from build123d import *

# Parameters (mm, degrees)
BOSS_EXTRUDE1_DEPTH = 168.35
FILLET1_R           = 1
SKETCH2_R           = 1.8
CUT_EXTRUDE1_DEPTH  = 200
CUT_EXTRUDE2_DEPTH  = 2
LPATTERN1_COUNT     = 3
LPATTERN1_PITCH     = 116
CUT_EXTRUDE3_DEPTH  = 1


with BuildPart() as part:
    # Sketch1 → Boss-Extrude1 (new body)
    with BuildSketch(Plane.XY):
        Polygon((0, 0), (5.8, 0), (8.7, 3.9), (-2.9, 3.9), align=None)
    extrude(amount=BOSS_EXTRUDE1_DEPTH)

    # Fillet1
    fillet1_edges = [part.edges().sort_by_distance(p)[0] for p in [
        (-2.9, 3.9, 84.175),
        (8.7, 3.9, 84.175),
    ]]
    fillet(fillet1_edges, radius=FILLET1_R)

    # Sketch2 → Cut-Extrude1 (cut)
    with BuildSketch(Plane.XZ):
        with Locations(Location((2.9, 126, 0), (0, 0, 270))):
            Circle(SKETCH2_R)
    cut_extrude1 = extrude(amount=-CUT_EXTRUDE1_DEPTH, mode=Mode.SUBTRACT)

    # Sketch3 → Cut-Extrude2 (cut)
    with BuildSketch(Plane.XZ):
        Polygon((2.902268292, 122.651369207), (5.80113348, 124.327649002), (5.798865189, 127.676279795), (2.897731708, 129.348630793), (-0.00113348, 127.672350998), (0.001134811, 124.323720205), align=None)
    cut_extrude2 = extrude(amount=-CUT_EXTRUDE2_DEPTH, mode=Mode.SUBTRACT)

    # LPattern1: Cut-Extrude1, Cut-Extrude2 ×3
    with Locations(*[(0, 0, -i * LPATTERN1_PITCH) for i in range(1, LPATTERN1_COUNT)]):
        add(cut_extrude1, mode=Mode.SUBTRACT)
        add(cut_extrude2, mode=Mode.SUBTRACT)

    # Sketch4 → Cut-Extrude3 (cut)
    with BuildSketch(Plane(origin=(0, 3.9, 0), x_dir=(1, 0, 0), z_dir=(0, 1, 0))):
        with BuildLine():
            Line((5.439754142, -74.65), (5.439754142, -75.626923077))
            Line((5.439754142, -75.626923077), (2.199880343, -75.626923077))
            Line((2.199880343, -75.626923077), (1.686614118, -78.132196514))
            add(Edge.make_bspline(
                [(1.686614118, -78.132196514), (1.787459033, -78.10435556), (1.982830106, -78.050418115), (2.271192299, -77.990530983), (2.544946796, -77.954430025), (2.722589054, -77.949500672), (2.808549214, -77.947115385)],
                knots=[0, 0, 0, 0, 1.100273476, 2.13160584, 3.095893838, 4, 4, 4, 4], degree=3))
            add(Edge.make_bspline(
                [(2.808549214, -77.947115385), (2.91491282, -77.949417538), (3.124050244, -77.953944147), (3.430044807, -77.997410395), (3.722143609, -78.065826877), (3.999735773, -78.161404868), (4.263334843, -78.283623499), (4.510515564, -78.43629548), (4.74498817, -78.614639759), (4.96254623, -78.819685828), (5.159915954, -79.045351085), (5.33345054, -79.287987862), (5.480850161, -79.545238143), (5.599397644, -79.819559799), (5.694060725, -80.107920067), (5.757067225, -80.413353024), (5.799022697, -80.732979693), (5.803710049, -80.951522845), (5.806100295, -81.062965745)],
                knots=[0, 0, 0, 0, 1.052922333, 2.070308379, 3.05430497, 4.020497103, 4.973039431, 5.925935799, 6.892292201, 7.88610001, 8.88166317, 9.857072816, 10.836096531, 11.812156883, 12.81219415, 13.836441305, 14.89672472, 16, 16, 16, 16], degree=3))
            add(Edge.make_bspline(
                [(5.806100295, -81.062965745), (5.804290341, -81.140586931), (5.800694891, -81.294780318), (5.782410734, -81.52377275), (5.747207107, -81.747917317), (5.699942087, -81.967243755), (5.638594506, -82.181336832), (5.564329295, -82.390809347), (5.473444392, -82.594357527), (5.373754721, -82.793907352), (5.261505377, -82.984947575), (5.136922439, -83.163606603), (5.005299209, -83.332564541), (4.863672296, -83.490009343), (4.710725302, -83.634906413), (4.548310535, -83.768115664), (4.377723993, -83.891889856), (4.196326512, -84.00120473), (4.008160183, -84.101796775), (3.810507678, -84.184320116), (3.6078682, -84.258099482), (3.397325217, -84.316908268), (3.179355627, -84.362989005), (2.953600131, -84.394287068), (2.721242736, -84.417082945), (2.563740024, -84.418509945), (2.484180223, -84.419230769)],
                knots=[0, 0, 0, 0, 1.056347294, 2.098418968, 3.122841568, 4.141288669, 5.149314143, 6.15115421, 7.162517403, 8.180376062, 9.185164535, 10.17417709, 11.141909838, 12.097768115, 13.052685741, 14.0056014, 14.954263652, 15.917497458, 16.885230207, 17.854509472, 18.828990115, 19.81800267, 20.826176721, 21.857883937, 22.917946725, 24, 24, 24, 24], degree=3))
            add(Edge.make_bspline(
                [(2.484180223, -84.419230769), (2.389272632, -84.417350703), (2.202553157, -84.413651895), (1.928993613, -84.374957303), (1.665791722, -84.319538359), (1.415066233, -84.236163939), (1.174570151, -84.131695658), (0.947541183, -83.999662363), (0.728178321, -83.850040659), (0.525399135, -83.673473413), (0.337195712, -83.48048145), (0.16872157, -83.271046726), (0.018679479, -83.048625887), (-0.110527818, -82.812138768), (-0.22074029, -82.562206766), (-0.307322508, -82.297893456), (-0.377204317, -82.020579874), (-0.40676834, -81.829662107), (-0.42178432, -81.732692308)],
                knots=[0, 0, 0, 0, 1.0467383, 2.05933395, 3.04377827, 4.011590433, 4.970194871, 5.932262533, 6.905835911, 7.896367577, 8.894135286, 9.877477877, 10.858688626, 11.851381753, 12.8477658, 13.868841284, 14.917554742, 16, 16, 16, 16], degree=3))
            Line((-0.42178432, -81.732692308), (0.433023372, -81.732692308))
            add(Edge.make_bspline(
                [(0.433023372, -81.732692308), (0.454056089, -81.823523939), (0.494482139, -81.998107378), (0.583216355, -82.243393385), (0.691708488, -82.461976416), (0.820716036, -82.656747924), (0.974612905, -82.826589553), (1.150225136, -82.977947414), (1.347114297, -83.114495445), (1.565898729, -83.228313118), (1.796711466, -83.325383083), (2.038285088, -83.390021624), (2.284041916, -83.435471911), (2.450262338, -83.440021489), (2.533789598, -83.442307692)],
                knots=[0, 0, 0, 0, 1.136247022, 2.183929868, 3.172523383, 4.106158343, 5.02341133, 5.958108904, 6.928429099, 7.938127109, 8.96079061, 9.975095812, 10.982467395, 12, 12, 12, 12], degree=3))
            add(Edge.make_bspline(
                [(2.533789598, -83.442307692), (2.615319365, -83.440074004), (2.775852142, -83.435675853), (3.01210313, -83.40182397), (3.240193881, -83.349688008), (3.457873759, -83.271665046), (3.668951949, -83.176837633), (3.868089138, -83.055148749), (4.061046254, -82.915103984), (4.241825675, -82.754657727), (4.40739589, -82.577847343), (4.553689334, -82.38876958), (4.675546506, -82.187065876), (4.778237188, -81.976228224), (4.856215094, -81.753945865), (4.911843764, -81.521260524), (4.944509231, -81.277597471), (4.9490028, -81.111401706), (4.951292603, -81.02671274)],
                knots=[0, 0, 0, 0, 1.027316725, 2.022795036, 3.002884548, 3.971462791, 4.93288096, 5.914575861, 6.907176829, 7.935150275, 8.956128384, 9.956726525, 10.942570165, 11.921478529, 12.907843606, 13.90538589, 14.932640048, 16, 16, 16, 16], degree=3))
            add(Edge.make_bspline(
                [(4.951292603, -81.02671274), (4.949500598, -80.950306588), (4.945993004, -80.800752415), (4.917334809, -80.581951718), (4.867486477, -80.374924367), (4.798297204, -80.17867063), (4.710450829, -79.993005405), (4.603100508, -79.817737077), (4.474231618, -79.655175717), (4.327024407, -79.505245267), (4.165757881, -79.366874572), (3.98765741, -79.248916737), (3.796450038, -79.149682789), (3.594439485, -79.064044879), (3.376820725, -79.002538565), (3.147903318, -78.956361677), (2.905215278, -78.929649869), (2.739287905, -78.925943587), (2.65399693, -78.924038462)],
                knots=[0, 0, 0, 0, 1.045622112, 2.046656509, 3.013763289, 3.955457236, 4.890082067, 5.820317437, 6.762574623, 7.722996705, 8.69280354, 9.665887285, 10.63943826, 11.638615906, 12.663482002, 13.728887084, 14.832589034, 16, 16, 16, 16], degree=3))
            add(Edge.make_bspline(
                [(2.65399693, -78.924038462), (2.580167488, -78.925618499), (2.427728421, -78.928880875), (2.193895585, -78.952901556), (1.948173111, -78.991652779), (1.691502948, -79.044955352), (1.423114279, -79.114708497), (1.143573489, -79.198295816), (0.85229282, -79.298232113), (0.656029585, -79.373703352), (0.555138757, -79.4125)],
                knots=[0, 0, 0, 0, 0.817624296, 1.688186739, 2.600797293, 3.572016777, 4.590301741, 5.671205678, 6.80286297, 8, 8, 8, 8], degree=3))
            Line((0.555138757, -79.4125), (1.532061834, -74.65))
            Line((1.532061834, -74.65), (5.439754142, -74.65))
        make_face()
    extrude(amount=-CUT_EXTRUDE3_DEPTH, mode=Mode.SUBTRACT)


solid = part.part
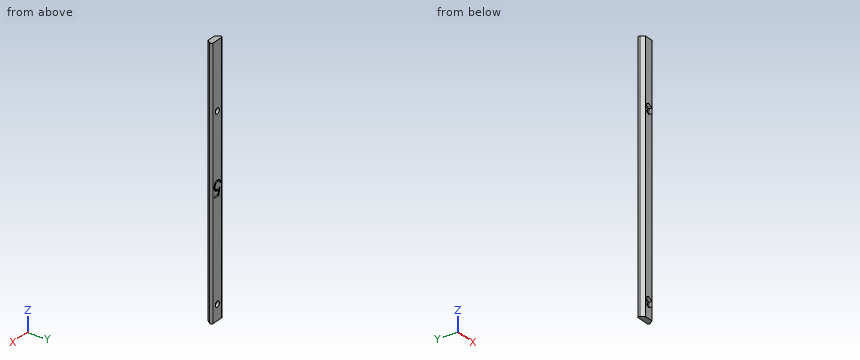
Geometry check sheet. Reference: the model listing, model coordinates, mm. Give positions to 0.01 mm unless a question says otherwise; leave off trailing zeros. Order: outer loops, then holes, each group sorted by start corner. A loop starts at its lowest first (then second) coordinate and runs counter-clockwise, first axis right, second up. Notation, with made-up numbers: M -2,79.25 L 47,79.25 A17 ccw 47,105.25 Z; hole C -17.5,58 d2. An arc over 180 degrees is marked long. Use a Markdown table: item, result.
Item 1: Material ranges on line 1 along Z through (x, y) = (4.25, 0.75); line 2 along Z through (x, y) = (2, 1.45); line 3 along X through (y, z) = (2.7, 21), recorded low to high.
Answers follow:
| item | result |
|---|---|
| line 1 | z = 0 to 7.43, 12.57 to 123.43, 128.57 to 168.35 |
| line 2 | z = 0 to 7.17, 12.83 to 123.17, 128.83 to 168.35 |
| line 3 | x = -1.89 to 7.69 |
Item 2: Section check B-B (y = 0.8). Record the cut outline in (x, z), and give its area (3 significant figures).
Answers follow:
| item | result |
|---|---|
| outline | M -0.59,0 L 6.39,0 L 6.39,168.35 L -0.59,168.35 Z; hole M 0,8.32 L 2.9,6.65 L 5.8,8.33 L 5.8,11.68 L 2.9,13.35 L 0,11.67 Z; hole M 0,124.32 L 2.9,122.65 L 5.8,124.33 L 5.8,127.68 L 2.9,129.35 L 0,127.67 Z |
| area | 1,120 mm2 |
Item 3: Section check A-A (z = 120.5). Record the cut outline in (x, y), and give its area (3 significant figures).
Answers follow:
| item | result |
|---|---|
| outline | M -1.71,2.3 L 0,0 L 5.8,0 L 7.51,2.3 A1 ccw 6.71,3.9 L -0.91,3.9 A1 ccw Z |
| area | 32.2 mm2 |
Item 4: Depth check by flat-ended pin: P1, Ø2, axis at y = 1.5, z = 121, coming from the -X side. Enter the tip coordinate at first touch or a pass-through.
Answers follow:
| item | result |
|---|---|
| P1 | stops at x = -1.83 |
